```python
from build123d import *

# Parameters (mm, degrees)
SKETCH1_W                    = 59
SKETCH1_H                    = 30
BOSS_EXTRUDE1_DEPTH          = 30
SKETCH2_R                    = 2.5
SKETCH2_R_2                  = 3.5
CUT_EXTRUDE1_DEPTH           = 52.674461778
SKETCH3_W                    = 59
SKETCH3_H                    = 60
BOSS_EXTRUDE2_DEPTH          = 30
FILLET2_R                    = 5
FILLET3_R                    = 5
SKETCH5_W                    = 59
SKETCH5_H                    = 90
BOSS_EXTRUDE3_DEPTH          = 120
SKETCH6_W                    = 75.4
SKETCH6_H                    = 6.2
CUT_EXTRUDE2_DEPTH           = 120
SKETCH6_3_W                  = 49.48
SKETCH6_3_H                  = 50
BOSS_EXTRUDE4_DEPTH          = 10
F_5_0_5_DIAMETER_HOLE1_D     = 5
F_5_0_5_DIAMETER_HOLE1_DEPTH = 18.497848452
F_5_0_5_DIAMETER_HOLE1_TIP   = 1.502151548
SKETCH14_W                   = 49.48
SKETCH14_H                   = 50
BOSS_EXTRUDE6_DEPTH          = 10
F_5_0_5_DIAMETER_HOLE2_D     = 5
F_5_0_5_DIAMETER_HOLE2_DEPTH = 18.497848452
F_5_0_5_DIAMETER_HOLE2_TIP   = 1.502151548
FILLET4_R                    = 1
FILLET5_R                    = 1
FILLET6_R                    = 1
FILLET7_R                    = 1
FILLET8_R                    = 1
FILLET9_R                    = 1
FILLET10_R                   = 1
FILLET11_R                   = 1
F_5_0_5_DIAMETER_HOLE3_D     = 5
F_5_0_5_DIAMETER_HOLE3_DEPTH = 18.497848452
F_5_0_5_DIAMETER_HOLE3_TIP   = 1.502151548
CUT_EXTRUDE3_START           = -75
SKETCH21_R                   = 2.35
CUT_EXTRUDE3_DEPTH           = 20


with BuildPart() as part:
    # Sketch1 → Boss-Extrude1 (new body)
    with BuildSketch(Plane.XY):
        Rectangle(SKETCH1_W, SKETCH1_H)
        Polygon((4, 2.727207794), (6.572792206, 5.3), (8, 5.3), (8, 3.1), (10, 5.1), (10, 10), (5.1, 10), (3.1, 8), (5.3, 8), (5.3, 6.572792206), (2.727207794, 4), (-2.727207794, 4), (-5.3, 6.572792206), (-5.3, 8), (-3.1, 8), (-5.1, 10), (-10, 10), (-10, 5.1), (-8, 3.1), (-8, 5.3), (-6.572792206, 5.3), (-4, 2.727207794), (-4, -2.727207794), (-6.572792206, -5.3), (-8, -5.3), (-8, -3.1), (-10, -5.1), (-10, -10), (-5.1, -10), (-3.1, -8), (-5.3, -8), (-5.3, -6.572792206), (-2.727207794, -4), (2.727207794, -4), (5.3, -6.572792206), (5.3, -8), (3.1, -8), (5.1, -10), (10, -10), (10, -5.1), (8, -3.1), (8, -5.3), (6.572792206, -5.3), (4, -2.727207794), align=None, mode=Mode.SUBTRACT)
    extrude(amount=-BOSS_EXTRUDE1_DEPTH)

    # Sketch2 → Cut-Extrude1 (cut, through all)
    with BuildSketch(Plane(origin=(0, 15, 0), x_dir=(1, 0, 0), z_dir=(0, 1, 0))):
        with Locations(Location((0, 10, 0), (0, 0, 270))):
            Circle(SKETCH2_R)
        with Locations(Location((0, 20, 0), (0, 0, 270))):
            Circle(SKETCH2_R)
        with Locations(Location((-23, 24.5, 0), (0, 0, 270))):
            Circle(SKETCH2_R_2)
        with Locations(Location((23, 24.5, 0), (0, 0, 270))):
            Circle(SKETCH2_R_2)
        with Locations(Location((23, 11.5, 0), (0, 0, 270))):
            Circle(SKETCH2_R_2)
        with Locations(Location((-23, 11.5, 0), (0, 0, 270))):
            Circle(SKETCH2_R_2)
    extrude(amount=-CUT_EXTRUDE1_DEPTH, mode=Mode.SUBTRACT)

    # Sketch3 → Boss-Extrude2 (add)
    with BuildSketch(Plane.XY):
        with Locations((0, -45)):
            Rectangle(SKETCH3_W, SKETCH3_H)
    extrude(amount=-BOSS_EXTRUDE2_DEPTH)

    # Fillet2
    fillet2_edges = [part.edges().sort_by_distance(p)[0] for p in [
        (29.5, -30, -30),
    ]]
    fillet(fillet2_edges, radius=FILLET2_R)

    # Fillet3
    fillet3_edges = [part.edges().sort_by_distance(p)[0] for p in [
        (-29.5, -30, -30),
    ]]
    fillet(fillet3_edges, radius=FILLET3_R)

    # Sketch5 → Boss-Extrude3 (add)
    with BuildSketch(Plane.XY):
        with Locations((0, -30)):
            Rectangle(SKETCH5_W, SKETCH5_H)
    extrude(amount=BOSS_EXTRUDE3_DEPTH)

    # Sketch6 → Cut-Extrude2 (cut)
    with BuildSketch(Plane.ZY.offset(29.5)):
        with Locations((82.3, 11.9)):
            Rectangle(SKETCH6_W, SKETCH6_H)
    extrude(amount=-CUT_EXTRUDE2_DEPTH, mode=Mode.SUBTRACT)

    # Sketch6<3> → Boss-Extrude4 (add)
    with BuildSketch(Plane.ZY.offset(29.5)):
        with Locations((19.86, 40)):
            Rectangle(SKETCH6_3_W, SKETCH6_3_H)
    extrude(amount=-BOSS_EXTRUDE4_DEPTH)

    # Ø5.0 (5) Diameter Hole1
    with Locations(Plane.XY.offset(44.6)):
        with Locations((-23.56, 60.57)):
            Hole(F_5_0_5_DIAMETER_HOLE1_D / 2, depth=F_5_0_5_DIAMETER_HOLE1_DEPTH)
            with Locations((0, 0, -(F_5_0_5_DIAMETER_HOLE1_DEPTH + F_5_0_5_DIAMETER_HOLE1_TIP / 2))):  # 118° drill point
                Cone(0, F_5_0_5_DIAMETER_HOLE1_D / 2, F_5_0_5_DIAMETER_HOLE1_TIP, mode=Mode.SUBTRACT)

    # Sketch14 → Boss-Extrude6 (add)
    with BuildSketch(Plane(origin=(29.5, 0, 0), x_dir=(0, 0, -1), z_dir=(1, 0, 0))):
        with Locations((-19.86, 40)):
            Rectangle(SKETCH14_W, SKETCH14_H)
    extrude(amount=-BOSS_EXTRUDE6_DEPTH)

    # Ø5.0 (5) Diameter Hole2
    with Locations(Plane.XY.offset(44.6)):
        with Locations((23.56, 60.57)):
            Hole(F_5_0_5_DIAMETER_HOLE2_D / 2, depth=F_5_0_5_DIAMETER_HOLE2_DEPTH)
            with Locations((0, 0, -(F_5_0_5_DIAMETER_HOLE2_DEPTH + F_5_0_5_DIAMETER_HOLE2_TIP / 2))):  # 118° drill point
                Cone(0, F_5_0_5_DIAMETER_HOLE2_D / 2, F_5_0_5_DIAMETER_HOLE2_TIP, mode=Mode.SUBTRACT)

    # Fillet4
    fillet4_edges = [part.edges().sort_by_distance(p)[0] for p in [
        (-29.5, 40, -4.88),
    ]]
    fillet(fillet4_edges, radius=FILLET4_R)

    # Fillet5
    fillet5_edges = [part.edges().sort_by_distance(p)[0] for p in [
        (-19.5, 40, -4.88),
    ]]
    fillet(fillet5_edges, radius=FILLET5_R)

    # Fillet6
    fillet6_edges = [part.edges().sort_by_distance(p)[0] for p in [
        (29.5, 40, -4.88),
    ]]
    fillet(fillet6_edges, radius=FILLET6_R)

    # Fillet7
    fillet7_edges = [part.edges().sort_by_distance(p)[0] for p in [
        (19.5, 40, -4.88),
    ]]
    fillet(fillet7_edges, radius=FILLET7_R)

    # Fillet8
    fillet8_edges = [part.edges().sort_by_distance(p)[0] for p in [
        (-19.5, 65, 20.36),
        (-29.5, 65, 20.36),
        (-29.207106781, 65, -4.587106781),
        (-24.5, 65, -4.88),
        (-19.792893219, 65, -4.587106781),
    ]]
    fillet(fillet8_edges, radius=FILLET8_R)

    # Fillet9
    fillet9_edges = [part.edges().sort_by_distance(p)[0] for p in [
        (29.5, 65, 20.36),
        (29.207106781, 65, -4.587106781),
        (19.5, 65, 20.36),
        (24.5, 65, -4.88),
        (19.792893219, 65, -4.587106781),
    ]]
    fillet(fillet9_edges, radius=FILLET9_R)

    # Fillet10
    fillet10_edges = [part.edges().sort_by_distance(p)[0] for p in [
        (29.5, -33.1, 120),
    ]]
    fillet(fillet10_edges, radius=FILLET10_R)

    # Fillet11
    fillet11_edges = [part.edges().sort_by_distance(p)[0] for p in [
        (-29.5, -33.1, 120),
    ]]
    fillet(fillet11_edges, radius=FILLET11_R)

    # Ø5.0 (5) Diameter Hole3
    with Locations(Plane.XY.offset(44.6)):
        with Locations((-23.56, 13.43), (23.56, 13.43)):
            Hole(F_5_0_5_DIAMETER_HOLE3_D / 2, depth=F_5_0_5_DIAMETER_HOLE3_DEPTH)
            with Locations((0, 0, -(F_5_0_5_DIAMETER_HOLE3_DEPTH + F_5_0_5_DIAMETER_HOLE3_TIP / 2))):  # 118° drill point
                Cone(0, F_5_0_5_DIAMETER_HOLE3_D / 2, F_5_0_5_DIAMETER_HOLE3_TIP, mode=Mode.SUBTRACT)

    # Sketch21 → Cut-Extrude3 (cut)
    with BuildSketch(Plane(origin=(0, 0, 0), x_dir=(1, 0, 0), z_dir=(0, 1, 0)).offset(CUT_EXTRUDE3_START)):
        with Locations(Location((0, -70.33, 0), (0, 0, 90))):
            Circle(SKETCH21_R)
        with Locations(Location((0, -20.66, 0), (0, 0, 90))):
            Circle(SKETCH21_R)
    extrude(amount=CUT_EXTRUDE3_DEPTH, mode=Mode.SUBTRACT)


solid = part.part
```
The listing builds one solid part. Answer for the finished solid, in the listing's coordinates (mm). A direction names the side the tool comes from. Round coordinates to 2 decimals unless told otherwise and drop trailing zeros. Write each loop counter-clockwise with the first axis right and the second up, starting at its lowest first coordinate (ties: lowest second). Pieces come first, ordered by that corner, then holes. Notation, with made-up numbers: (86, 15.5) -> (124, 15.5) arc R36 cw to (124, 54.5) -> close; hole circle Ø2 at (-31.75, 27). An arc over 180 degrees is marked (long way). Answer as a JSON object with one key per item and string values. Group by question number.
Q1. Section C-C (z = 70.33) is taken. Write down the section's boundary in (x, y).
Q2. Straight lines are drawn through the part: line 1 along Y through (x, z) = (7, -18.5); line 2 along X through (y, z) = (13.43, 32); line 3 along X through (y, z) = (13, 35). For each, find the intervals that lie inside material, in ascending order.
Q3. Determine the mould class of faces 5 (the face through (0, -75, 44)), 6 (the face through (0.9, -65.14, 18.49)) for opening direction X: pulls with the +X half, pulls with the -X half, needs draft (parallel to the pull), parting line crosses it, or undercut.
Q4. Which of the six approach directions +Z, -Z, +X, -X, +Y, -Y give full straight-line access (tool end or side, diameter ignored) to faces 1 (the face through (0.1, -9.4, -12.5)), 2 (the face through (24.1, 58.13, 35.22)), 3 (the face through (19.5, 40, 21)), 4 (the face through (-8, 10, -15))?
Q5. Section B-B (x = 0) is taken. Count the separate pieces of the cut face and the enclosed holes in it, plus the area to 3 significant figures.
Q6. Section D-D (x = -16) is taken. Write down the section's boundary in (y, z), plus the area to 3 significant figures.
Q7. Each of these flat-tipped pins is pushed along its axis until it touches: pin 1 Ø0.7 at (x, z) = (-4.5, -18) entering from +Y; pin 2 Ø4 at (x, z) = (-1.5, 54) entering from +Y; pin 3 Ø1.4 at (x, z) = (-1, 70) entering from -Y. Where does it stop, or does it pass through?
Q8. Section A-A (y = 31.5) is taken. Write down the section's boundary in (x, z), plus the area to 3 significant figures.
Check values:
{
 "1": {"outline": "(-29.5, -75) -> (-2.35, -75) -> (-2.35, -55) -> (2.35, -55) -> (2.35, -75) -> (29.5, -75) -> (29.5, 8.8) -> (-29.5, 8.8) -> close"},
 "2": {"line 1": "-75 to -10, -5.3 to 5.3, 10 to 15", "line 2": "-29.5 to -26.06, -21.06 to 21.06, 26.06 to 29.5", "line 3": "-29.5 to -26.02, -21.1 to 21.1, 26.02 to 29.5"},
 "3": {"face 5": "needs draft", "face 6": "undercut"},
 "4": {"face 1": "+Y", "face 2": "+Z", "face 3": "+Z, -Z, +Y", "face 4": "-Z"},
 "5": {"separate pieces": "3", "enclosed holes": "0", "area": "12,400 mm^2"},
 "6": {"outline": "(-75, -30) -> (15, -30) -> (15, 44.6) -> (8.8, 44.6) -> (8.8, 120) -> (-75, 120) -> close", "area": "13,000 mm^2"},
 "7": {"pin 1": "y = 15", "pin 2": "y = 8.8", "pin 3": "y = -55"},
 "8": {"outline": "(-29.5, -3.88) arc R1 ccw to (-28.5, -4.88) -> (-20.5, -4.88) arc R1 ccw to (-19.5, -3.88) -> (-19.5, 44.6) -> (-29.5, 44.6) -> close; (19.5, -3.88) arc R1 ccw to (20.5, -4.88) -> (28.5, -4.88) arc R1 ccw to (29.5, -3.88) -> (29.5, 44.6) -> (19.5, 44.6) -> close", "area": "989 mm^2"}
}
